from build123d import *

# Parameters (mm, degrees)
SKETCH_1_W          = 8
SKETCH_1_H          = 15
EXTRUDE_1_DEPTH     = 5
SKETCH_2_W          = 8
SKETCH_2_H          = 5
EXTRUDE_2_DEPTH     = 45
EXTRUDE_3_DEPTH     = 8
CUT_EXTRUDE_1_DEPTH = 48.657633177
FILLET_1_R          = 20
FILLET_2_R          = 2
HOLE_WIZARD_M3_1_D  = 3.4


with BuildPart() as part:
    # ｽｹｯﾁ1 → ﾎﾞｽ - 押し出し1 (new body)
    with BuildSketch(Plane.XY):
        Rectangle(SKETCH_1_W, SKETCH_1_H)
    extrude(amount=EXTRUDE_1_DEPTH)

    # ｽｹｯﾁ2 → ﾎﾞｽ - 押し出し2 (add)
    with BuildSketch(Plane(origin=(0, 0, 0), x_dir=(-1, 0, 0), z_dir=(0, 0, -1))):
        with Locations((0, 5)):
            Rectangle(SKETCH_2_W, SKETCH_2_H)
    extrude(amount=EXTRUDE_2_DEPTH)

    # ｽｹｯﾁ4 → ﾎﾞｽ - 押し出し3 (add)
    with BuildSketch(Plane.ZY.offset(4)):
        Polygon((-45, 7.5), (-45, 13.5), (-42, 10.5), (-43, 10.5), (-43, 7.5), align=None)
        Polygon((-21.5, 7.5), (-21.5, 10.5), (-22.5, 10.5), (-19.5, 13.5), (-19.5, 7.5), align=None)
    extrude(amount=-EXTRUDE_3_DEPTH)

    # ｽｹｯﾁ5 → ｶｯﾄ - 押し出し1 (cut, through all)
    with BuildSketch(Plane.ZY.offset(4)):
        Polygon((-45, 2.5), (-45, 5.5), (-15, 5.5), (-3.803847577, 2.5), align=None)
    extrude(amount=-CUT_EXTRUDE_1_DEPTH, mode=Mode.SUBTRACT)

    # ﾌｨﾚｯﾄ1
    fillet_1_edges = [part.edges().sort_by_distance(p)[0] for p in [
        (0, 2.5, -3.803847577),
        (0, 5.5, -15),
    ]]
    fillet(fillet_1_edges, radius=FILLET_1_R)

    # ﾌｨﾚｯﾄ2
    fillet_2_edges = [part.edges().sort_by_distance(p)[0] for p in [
        (0, 2.5, 0),
    ]]
    fillet(fillet_2_edges, radius=FILLET_2_R)

    # M3 すきま穴1 (through all)
    with Locations(Plane.XY.offset(5)):
        with Locations((0, -4.5)):
            Hole(HOLE_WIZARD_M3_1_D / 2)


solid = part.part
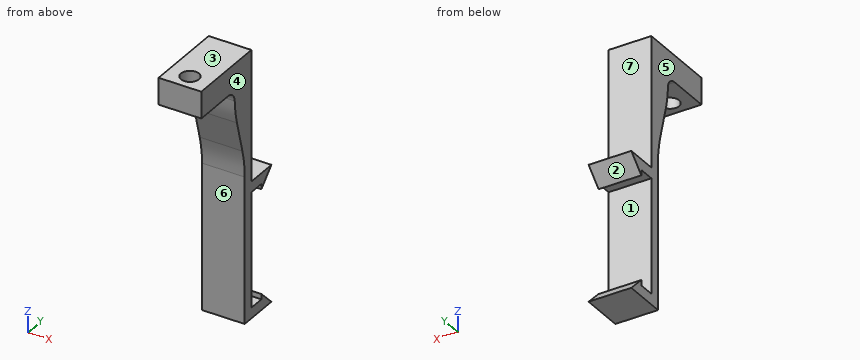
Geometry check sheet. Reference: the model listing, model coordinates, mm. Face numbers are marked on the shaded views. A direction names the side the tool comes from. Give positions to 0.01 mm unless a question says otherwise; leave off trailing zeros. Order: outer loops, then holes, each group sorted by start corner. A loop starts at its lowest first (then second) coordinate and runs counter-clockwise, first axis right, second up.
1) Cross-section at B-B (z = 0.5). Record the boundary of the cut face in (x, y), then the cut area to 3 significant figures.
Results are:
outline: (-4, -7.5) - (4, -7.5) - (4, 7.5) - (-4, 7.5) - close; hole circle Ø3.4 at (0, -4.5)
area: 111 mm2
2) Material ranges on probe 1 along Y at (x, z) = (0, 2.25); probe 2 along Z at (x, y) = (1.25, 10.25); probe 3 along Z at (x, y) = (1.75, 11), recorded low to high.
Results are:
probe 1: y = -7.5 to -6.2, -2.8 to 7.5
probe 2: z = -45 to -43, -21.5 to -19.5
probe 3: z = -45 to -42.5, -22 to -19.5
3) Cross-section at A-A (y = -4.5). Record the boundary of the cut face in (x, z), then the cut area to 3 significant figures.
Results are:
outline: (-4, 0) - (-1.7, 0) - (-1.7, 5) - (-4, 5) - close; (1.7, 0) - (4, 0) - (4, 5) - (1.7, 5) - close
area: 23.0 mm2
4) Tool access check on the marked faces 5, 6 and 7. Record the directions out of +Z, -Z, +X, -X, +Y, -Y that give a thin tool (end or side, any length) a straight path to the whole face; none if there is none.
Results are:
face 5: +Z, -Z, -X, +Y, -Y
face 6: -Z, +X, -X, -Y
face 7: +Z, +X, -X, +Y
5) Gauge pin test, flat ends, axial feed: pin 1 (1.5 mm diameter, centred on x = 1.5, z = -33, fed in from -Y); pin 2 (0.9 mm diameter, centred on x = -1, y = 9, fed in from +Z); pin 3 (2.5 mm diameter, centred on x = -1.5, y = -2.5, fed in from -Z). Record the tip position at first contact, or that the pin passes through.
Results are:
pin 1: stops at y = 5.5
pin 2: stops at z = -19.5
pin 3: stops at z = 0
6) Draft check along Z on the marked faces 1, 2, 3 and 4. Enter one of: released by +Z, released by -Z, zero draft, split by the parting line, or undercut.
Results are:
face 1: undercut
face 2: undercut
face 3: released by +Z
face 4: zero draft
7) Cross-section at D-D (z = -32). Record the boundary of the cut face in (x, y).
Results are:
outline: (-4, 5.5) - (4, 5.5) - (4, 7.5) - (-4, 7.5) - close
8) Cross-section at C-C (y = 11.5). Record the boundary of the cut face in (x, z), then the cut area to 3 significant figures.
Results are:
outline: (-4, -45) - (4, -45) - (4, -43) - (-4, -43) - close; (-4, -21.5) - (4, -21.5) - (4, -19.5) - (-4, -19.5) - close
area: 32.0 mm2
